Design review of the part built by this model. Coordinates are the model's own, in mm. A direction names the side the tool comes from. Coordinates: 2 decimals unless noted, no trailing zeros. Loops run counter-clockwise (first coordinate to the right, second up) from the corner with the lowest first, then second, coordinate; pieces in that order, holes last. Notation, with made-up numbers: (20.5, 53) - (38.5, 53) arc R20 ccw to (38.5, 82) - close; hole circle Ø10 at (89.5, 32.5). An arc over 180 degrees is marked (long way). Return JSON: item names as keys, results as strings. Group by question number.
from build123d import *

# Parameters (mm, degrees)
SKETCH_1_R          = 5.75
EXTRUDE_1_DEPTH     = 9.25
FILLET_1_R          = 15
SKETCH_2_R          = 12.5
CUT_EXTRUDE_1_DEPTH = 3
SKETCH_3_R          = 2.1
CUT_EXTRUDE_2_DEPTH = 7.25
SKETCH_4_R          = 1
CUT_EXTRUDE_3_DEPTH = 7.25
SKETCH_5_R          = 9
SKETCH_5_R_2        = 5.75
EXTRUDE_2_DEPTH     = 8.75
SKETCH_6_R          = 4.71
SKETCH_6_R_2        = 2.1
EXTRUDE_3_DEPTH     = 2.5
CHAMFER_1_SIZE      = 0.5
CHAMFER_2_SIZE      = 0.5
SKETCH_7_R          = 3
CUT_EXTRUDE_4_DEPTH = 19


with BuildPart() as part:
    # ｽｹｯﾁ1 → ﾎﾞｽ - 押し出し1 (new body)
    with BuildSketch(Plane(origin=(0, 0, 0), x_dir=(1, 0, 0), z_dir=(0, 1, 0))):
        with BuildLine():
            Line((-8.324355962, -34.418207467), (5.773502692, -10))
            Line((5.773502692, -10), (33.96922, -10))
            ThreePointArc((33.96922, -10), (43.96922, 0), (33.96922, 10))
            Line((33.96922, 10), (5.773502692, 10))
            Line((5.773502692, 10), (-8.324355962, 34.418207467))
            ThreePointArc((-8.324355962, 34.418207467), (-21.98461, 38.078461505), (-25.644864038, 24.418207467))
            Line((-25.644864038, 24.418207467), (-11.547005384, 0))
            Line((-11.547005384, 0), (-25.644864038, -24.418207467))
            ThreePointArc((-25.644864038, -24.418207467), (-21.98461, -38.078461505), (-8.324355962, -34.418207467))
        make_face()
        with Locations((-16.98461, 29.418207467)):
            Circle(SKETCH_1_R, mode=Mode.SUBTRACT)
        with Locations((-16.98461, -29.418207467)):
            Circle(SKETCH_1_R, mode=Mode.SUBTRACT)
        with Locations((33.96922, 0)):
            Circle(SKETCH_1_R, mode=Mode.SUBTRACT)
    extrude(amount=EXTRUDE_1_DEPTH)

    # ﾌｨﾚｯﾄ1
    fillet_1_edges = [part.edges().sort_by_distance(p)[0] for p in [
        (5.773502692, 4.625, 10),
        (-11.547005384, 4.625, 0),
        (5.773502692, 4.625, -10),
    ]]
    fillet(fillet_1_edges, radius=FILLET_1_R)

    # ｽｹｯﾁ2 → ｶｯﾄ - 押し出し1 (cut)
    with BuildSketch(Plane(origin=(0, 9.25, 0), x_dir=(1, 0, 0), z_dir=(0, 1, 0))):
        Circle(SKETCH_2_R)
    extrude(amount=-CUT_EXTRUDE_1_DEPTH, mode=Mode.SUBTRACT)

    # ｽｹｯﾁ3 → ｶｯﾄ - 押し出し2 (cut, through all)
    with BuildSketch(Plane(origin=(0, 6.25, 0), x_dir=(1, 0, 0), z_dir=(0, 1, 0))):
        Circle(SKETCH_3_R)
    extrude(amount=-CUT_EXTRUDE_2_DEPTH, mode=Mode.SUBTRACT)

    # ｽｹｯﾁ4 → ｶｯﾄ - 押し出し3 (cut, through all)
    with BuildSketch(Plane(origin=(0, 6.25, 0), x_dir=(1, 0, 0), z_dir=(0, 1, 0))):
        with Locations((10, 0)):
            Circle(SKETCH_4_R)
        with Locations((8.090169944, -5.877852523)):
            Circle(SKETCH_4_R)
        with Locations((3.090169944, -9.510565163)):
            Circle(SKETCH_4_R)
        with Locations((-3.090169944, -9.510565163)):
            Circle(SKETCH_4_R)
        with Locations((-8.090169944, -5.877852523)):
            Circle(SKETCH_4_R)
        with Locations((-10, 0)):
            Circle(SKETCH_4_R)
        with Locations((-8.090169944, 5.877852523)):
            Circle(SKETCH_4_R)
        with Locations((-3.090169944, 9.510565163)):
            Circle(SKETCH_4_R)
        with Locations((3.090169944, 9.510565163)):
            Circle(SKETCH_4_R)
        with Locations((8.090169944, 5.877852523)):
            Circle(SKETCH_4_R)
    extrude(amount=-CUT_EXTRUDE_3_DEPTH, mode=Mode.SUBTRACT)

    # ｽｹｯﾁ5 → ﾎﾞｽ - 押し出し2 (add)
    with BuildSketch(Plane.XZ):
        with Locations((-16.98461, -29.418207467)):
            Circle(SKETCH_5_R)
        with Locations((-16.98461, -29.418207467)):
            Circle(SKETCH_5_R_2, mode=Mode.SUBTRACT)
        with Locations((-16.98461, 29.418207467)):
            Circle(SKETCH_5_R)
        with Locations((-16.98461, 29.418207467)):
            Circle(SKETCH_5_R_2, mode=Mode.SUBTRACT)
        with Locations((33.96922, 0)):
            Circle(SKETCH_5_R)
        with Locations((33.96922, 0)):
            Circle(SKETCH_5_R_2, mode=Mode.SUBTRACT)
    extrude(amount=EXTRUDE_2_DEPTH)

    # ｽｹｯﾁ6 → ﾎﾞｽ - 押し出し3 (add)
    with BuildSketch(Plane.XZ):
        Circle(SKETCH_6_R)
        Circle(SKETCH_6_R_2, mode=Mode.SUBTRACT)
    extrude(amount=EXTRUDE_3_DEPTH)

    # 面取り1
    chamfer_1_edges = [part.edges().sort_by_distance(p)[0] for p in [
        (-20.76099822, 0, -15.959103733),
        (-21.98461, 0, -38.078461505),
        (24.201488365, 0, -10),
        (43.96922, 0, 0),
        (-20.76099822, 0, 15.959103733),
        (-3.440490145, 0, -25.959103733),
        (24.201488365, 0, 10),
        (-13.867513459, 0, 0),
        (6.93375673, 0, -12.009618943),
        (6.93375673, 0, 12.009618943),
        (-3.440490145, 0, 25.959103733),
        (-21.98461, 0, 38.078461505),
    ]]
    chamfer(chamfer_1_edges, length=CHAMFER_1_SIZE)

    # 面取り2
    chamfer_2_edges = [part.edges().sort_by_distance(p)[0] for p in [
        (-21.98461, 9.25, -38.078461505),
        (-20.76099822, 9.25, -15.959103733),
        (-21.98461, 9.25, 38.078461505),
        (-3.440490145, 9.25, 25.959103733),
        (-20.76099822, 9.25, 15.959103733),
        (43.96922, 9.25, 0),
        (-3.440490145, 9.25, -25.959103733),
        (24.201488365, 9.25, 10),
        (-13.867513459, 9.25, 0),
        (6.93375673, 9.25, -12.009618943),
        (6.93375673, 9.25, 12.009618943),
        (24.201488365, 9.25, -10),
    ]]
    chamfer(chamfer_2_edges, length=CHAMFER_2_SIZE)

    # ｽｹｯﾁ7 → ｶｯﾄ - 押し出し4 (cut, through all)
    with BuildSketch(Plane(origin=(0, 9.25, 0), x_dir=(1, 0, 0), z_dir=(0, 1, 0))):
        with Locations((20, 0)):
            Circle(SKETCH_7_R)
        with Locations((-10, -17.320508076)):
            Circle(SKETCH_7_R)
        with Locations((-10, 17.320508076)):
            Circle(SKETCH_7_R)
    extrude(amount=-CUT_EXTRUDE_4_DEPTH, mode=Mode.SUBTRACT)


solid = part.part
Item 1: Add section B-B (y = -1). State the section outline as (x, z) points, then the cut area to 3 significant figures.
Item 2: For faces 5 (the face through (2.873, 3.169, 10.487)), 6 (the face through (-20.616, 8.996, -16.201)), 7 (the face through (-20.61, 0.25, -16.2)), 8 (the face through (24.98, -4.31, 0.4)), 9 (the face through (43.609, 9.108, 0.212)), list the 3-axis set-ups (+Z, -Z, +X, -X, +Y, -Y) from which the entire face can be reached by the end or side of a thin tool; tool diameter is ignored.
Item 3: Draft analysis for pull direction X (two halves, no side actions). For faces 1 (the face through (9.044, 3.169, 5.577)), 2 (the face through (-10.65, 4.69, 20.25)), 3 (the face through (-13.73, 8.89, -0.11)), 4 (the face through (-3.592, 0.247, -25.714)), state which applies: pulls with the +X half, pulls with the -X half, needs draft (parallel to the pull), parting line crosses it, or undercut.
Item 4: For P1, Ø10, axis at y = 2.5, z = -11.5, coming from the -X side; P2, Ø2.5, axis at x = -3.09, z = 9.51, coming from the -Y side; P3, Ø22.5, axis at x = 0, z = 0, coming from the +Y side; P4, Ø5, axis at x = -14.5, y = 1.5, coming from the +Z side, all flat-tipped, find the tip position at first contact; note any pin that passes through.
Item 5: Add section A-A (x = 20). State the section outline as (y, z) points, then the cut area to 3 significant figures.
Item 6: To check wall thickness, follow line 1 (X direction, y = 5, z = 0); line 2 (X direction, y = 7.3, z = 0); line 3 (Z direction, x = -19.5, y = 1.75) (3 decimals). State the ranges of each line that lie inside material, in increasing order. Write a range as from..to.
Item 7: Add section D-D (x = 0). State the section outline as (y, z) points.
Item 8: Add section C-C (z = 0). Give the number of separate pieces and of enclosed holes in the cut face, then the cut area to 3 significant figures.
Answers below:
{
 "1": {"outline": "circle Ø18 at (-16.98, -29.42); circle Ø18 at (-16.98, 29.42); circle Ø9.42 at (0, 0); circle Ø18 at (33.97, 0); hole circle Ø11.5 at (-16.98, -29.42); hole circle Ø11.5 at (-16.98, 29.42); hole circle Ø4.2 at (0, 0); hole circle Ø11.5 at (33.97, 0)", "area": "508 mm^2"},
 "2": {"face 5": "+Y, -Y", "face 6": "-X, +Y", "face 7": "-X, -Y", "face 8": "-Y", "face 9": "+X, +Y"},
 "3": {"face 1": "undercut", "face 2": "undercut", "face 3": "pulls with the -X half", "face 4": "pulls with the +X half"},
 "4": {"P1": "stops at x = -21.07", "P2": "stops at y = 0", "P3": "stops at y = 6.25", "P4": "stops at z = 39.42"},
 "5": {"outline": "(0, -9.5) - (0.5, -10) - (8.75, -10) - (9.25, -9.5) - (9.25, -3) - (0, -3) - close; (0, 3) - (9.25, 3) - (9.25, 9.5) - (8.75, 10) - (0.5, 10) - (0, 9.5) - close", "area": "129 mm^2"},
 "6": {"line 1": "x = -13.87..-11, -9..-2.1, 2.1..9, 11..17, 23..28.22, 39.72..43.97", "line 2": "x = -13.87..-12.5, 12.5..17, 23..28.22, 39.72..43.97", "line 3": "z = -39.097..-34.589, -24.248..-13.775, 13.775..24.248, 34.589..39.097"},
 "7": {"outline": "(-2.5, -4.71) - (0, -4.71) - (0, -19) - (0.5, -20) - (8.75, -20) - (9.25, -19) - (9.25, -12.5) - (6.25, -12.5) - (6.25, -2.1) - (-2.5, -2.1) - close; (-2.5, 2.1) - (6.25, 2.1) - (6.25, 12.5) - (9.25, 12.5) - (9.25, 19) - (8.75, 20) - (0.5, 20) - (0, 19) - (0, 4.71) - (-2.5, 4.71) - close"},
 "8": {"separate pieces": "6", "enclosed holes": "0", "area": "316 mm^2"}
}
